Input: part model. Units: mm. Frame: model coordinates. Face numbers are marked on the shaded views. A direction names the side the tool comes from. Coordinates: 2 decimals unless noted, no trailing zeros. Order: outer loops, then holes, each group sorted by start corner. A loop starts at its lowest first (then second) coordinate and runs counter-clockwise, first axis right, second up. Notation, with made-up numbers: (-3.75, 24) -> (22.25, 24) arc R21 cw to (22.25, 36) -> close; hole circle Ø6 at (22, 6.25). An arc over 180 degrees is marked (long way). One line per item, written item: value. Start each with the question number.
from build123d import *

# Parameters (mm, degrees)
SKETCH_1_W               = 90
SKETCH_1_H               = 90
EXTRUDE_2_DEPTH          = 45
SKETCH_2_W               = 80
SKETCH_2_H               = 80
CUT_EXTRUDE_1_DEPTH      = 40
EXTRUDE_3_DEPTH          = 10
SKETCH_4_R               = 1
EXTRUDE_4_DEPTH          = 2
SKETCH_5_R               = 6
CUT_EXTRUDE_2_DEPTH      = 30
EXTRUDE_5_DEPTH          = 6
CUT_EXTRUDE_START        = -2
CUT_EXTRUDE_3_DEPTH      = 6
SKETCH_8_R               = 12.5
CUT_EXTRUDE_4_DEPTH      = 6
SKETCH_9_R               = 6
CUT_EXTRUDE_5_DEPTH      = 6
SKETCH_10_R              = 2
EXTRUDE_6_DEPTH          = 5
CUT_EXTRUDE_6_DEPTH      = 86.341501801
CUT_EXTRUDE_6_DEPTH_BACK = 86.341501801
EXTRUDE_8_DEPTH          = 5
EXTRUDE_9_REACH          = 89.762
SKETCH_13_W              = 70
SKETCH_13_H              = 5
SKETCH_14_R              = 2
SKETCH_14_W              = 3.535716984
SKETCH_14_H              = 8
EXTRUDE_10_DEPTH         = 5


with BuildPart() as part:
    # 草图1 → 凸台-拉伸2 (new body)
    with BuildSketch(Plane.XY):
        Rectangle(SKETCH_1_W, SKETCH_1_H)
    extrude(amount=EXTRUDE_2_DEPTH)

    # 草图2 → 切除-拉伸1 (cut)
    with BuildSketch(Plane.XY.offset(45)):
        Rectangle(SKETCH_2_W, SKETCH_2_H)
    extrude(amount=-CUT_EXTRUDE_1_DEPTH, mode=Mode.SUBTRACT)

    # 草图3 → 凸台-拉伸3 (add)
    with BuildSketch(Plane(origin=(0, 45, 0), x_dir=(1, 0, 0), z_dir=(0, 1, 0))):
        with BuildLine():
            Line((-15.725, -45), (15.725, -45))
            ThreePointArc((15.725, -45), (0, -29.275), (-15.725, -45))
        make_face()
    extrude(amount=EXTRUDE_3_DEPTH)

    # 草图4 → 凸台-拉伸4 (add)
    with BuildSketch(Plane(origin=(0, 55, 0), x_dir=(1, 0, 0), z_dir=(0, 1, 0))):
        with BuildLine():
            Line((-13.344644505, -28.920245738), (13.344644505, -28.920245738))
            ThreePointArc((13.344644505, -28.920245738), (16.17307163, -30.091818614), (17.344644505, -32.920245738))
            Line((17.344644505, -32.920245738), (17.344644505, -45))
            Line((17.344644505, -45), (-17.344644505, -45))
            Line((-17.344644505, -45), (-17.344644505, -32.920245738))
            ThreePointArc((-17.344644505, -32.920245738), (-16.17307163, -30.091818614), (-13.344644505, -28.920245738))
        make_face()
        with Locations(Location((13.344644505, -32.920245738, 0), (0, 0, 270))):
            Circle(SKETCH_4_R, mode=Mode.SUBTRACT)
        with Locations(Location((-13.344644505, -32.920245738, 0), (0, 0, 270))):
            Circle(SKETCH_4_R, mode=Mode.SUBTRACT)
    extrude(amount=-EXTRUDE_4_DEPTH)

    # 草图5 → 切除-拉伸2 (cut)
    with BuildSketch(Plane(origin=(0, 55, 0), x_dir=(1, 0, 0), z_dir=(0, 1, 0))):
        with Locations((0, -45)):
            Circle(SKETCH_5_R)
    extrude(amount=-CUT_EXTRUDE_2_DEPTH, mode=Mode.SUBTRACT)

    # 草图6 → 凸台-拉伸5 (add)
    with BuildSketch(Plane.ZY.offset(45)):
        with BuildLine():
            Line((45.073955752, 16.4), (45.073955752, -13.6))
            ThreePointArc((45.073955752, -13.6), (30.073955752, 1.4), (45.073955752, 16.4))
        make_face()
    extrude(amount=EXTRUDE_5_DEPTH)

    # 草图7 → 切除-拉伸3 (cut)
    with BuildSketch(Plane(origin=(0, 55, 0), x_dir=(1, 0, 0), z_dir=(0, 1, 0)).offset(CUT_EXTRUDE_START)):
        with BuildLine():
            Line((-12.5, -45), (12.5, -45))
            ThreePointArc((12.5, -45), (0, -32.5), (-12.5, -45))
        make_face()
    extrude(amount=-CUT_EXTRUDE_3_DEPTH, mode=Mode.SUBTRACT)

    # 草图8 → 切除-拉伸4 (cut)
    with BuildSketch(Plane.ZY.offset(51)):
        with Locations((45.073955752, 1.4)):
            Circle(SKETCH_8_R)
    extrude(amount=-CUT_EXTRUDE_4_DEPTH, mode=Mode.SUBTRACT)

    # 草图9 → 切除-拉伸5 (cut)
    with BuildSketch(Plane.ZY.offset(45)):
        with Locations((45, 1.4)):
            Circle(SKETCH_9_R)
    extrude(amount=-CUT_EXTRUDE_5_DEPTH, mode=Mode.SUBTRACT)

    # 草图10 → 凸台-拉伸6 (add)
    # profile 1 of 4: a face of its own
    with BuildSketch(Plane.XY.offset(45)):
        with BuildLine():
            Line((-47.5, 45), (-42.902808048, 45))
            Line((-42.902808048, 45), (-42.902808048, 37))
            Line((-42.902808048, 37), (-47.5, 37))
            ThreePointArc((-47.5, 37), (-51.5, 41), (-47.5, 45))
        make_face()
        with Locations((-47.5, 41)):
            Circle(SKETCH_10_R, mode=Mode.SUBTRACT)
    # profile 2 of 4: a face of its own
    with BuildSketch(Plane.XY.offset(45)):
        with BuildLine():
            Line((-47.5, -45), (-42.902808048, -45))
            Line((-42.902808048, -45), (-42.902808048, -37))
            Line((-42.902808048, -37), (-47.5, -37))
            ThreePointArc((-47.5, -37), (-51.5, -41), (-47.5, -45))
        make_face()
        with Locations((-47.5, -41)):
            Circle(SKETCH_10_R, mode=Mode.SUBTRACT)
    # profile 3 of 4: a face of its own
    with BuildSketch(Plane.XY.offset(45)):
        with BuildLine():
            Line((42.460881889, 45), (42.460881889, 37))
            Line((42.460881889, 37), (47.5, 37))
            ThreePointArc((47.5, 37), (51.5, 41), (47.5, 45))
            Line((47.5, 45), (42.460881889, 45))
        make_face()
        with Locations((47.5, 41)):
            Circle(SKETCH_10_R, mode=Mode.SUBTRACT)
    # profile 4 of 4: a face of its own
    with BuildSketch(Plane.XY.offset(45)):
        with BuildLine():
            Line((41.065096799, -37), (41.065096799, -45))
            Line((41.065096799, -45), (47.5, -45))
            ThreePointArc((47.5, -45), (51.5, -41), (47.5, -37))
            Line((47.5, -37), (41.065096799, -37))
        make_face()
        with Locations((47.5, -41)):
            Circle(SKETCH_10_R, mode=Mode.SUBTRACT)
    extrude(amount=-EXTRUDE_6_DEPTH)

    # 草图11 → 切除-拉伸6 (cut, two sides: drawn at the far end of the back side and taken through both)
    with BuildSketch(Plane.XY.offset(5).offset(-CUT_EXTRUDE_6_DEPTH_BACK)):
        Polygon((25, 25), (25, 60.762211799), (85.89289348, 60.762211799), (85.89289348, -73.939659246), (-86.710921037, -73.939659246), (-86.710921037, -25), (-25, -25), (25, -25), align=None)
    extrude(amount=CUT_EXTRUDE_6_DEPTH + CUT_EXTRUDE_6_DEPTH_BACK, mode=Mode.SUBTRACT)

    # 草图12 → 凸台-拉伸8 (add)
    with BuildSketch(Plane(origin=(25, 0, 0), x_dir=(0, 0, -1), z_dir=(1, 0, 0))):
        Polygon((-45, 40), (-45, -25), (-5, -25), (0, -25), (0, 45), (-45, 45), align=None)
    extrude(amount=-EXTRUDE_8_DEPTH)

    # 草图13 → 凸台-拉伸9 (add, up to next)
    with BuildSketch(Plane.XY.offset(45), mode=Mode.PRIVATE) as extrude_9_sk1:
        with Locations((-10, -22.5)):
            Rectangle(SKETCH_13_W, SKETCH_13_H)
    extrude_9_tool1 = extrude(extrude_9_sk1.sketch, amount=-EXTRUDE_9_REACH, mode=Mode.PRIVATE) - part.part
    add(extrude_9_tool1.solids().sort_by_distance((-10, -22.5, 45))[0])

    # 草图14 → 凸台-拉伸10 (add)
    # profile 1 of 5: a face of its own
    with BuildSketch(Plane.XY.offset(45)):
        with BuildLine():
            Line((27.5, 45), (25, 45))
            Line((25, 45), (25, 37))
            Line((25, 37), (27.5, 37))
            ThreePointArc((27.5, 37), (31.5, 41), (27.5, 45))
        make_face()
        with Locations((27.5, 41)):
            Circle(SKETCH_14_R, mode=Mode.SUBTRACT)
    # profile 2 of 5: a face of its own
    with BuildSketch(Plane.XY.offset(45)):
        with Locations((-43.232141508, -21)):
            Rectangle(SKETCH_14_W, SKETCH_14_H)
    # profile 3 of 5: a face of its own
    with BuildSketch(Plane.XY.offset(45)):
        with Locations((23.232141508, -21)):
            Rectangle(SKETCH_14_W, SKETCH_14_H)
    # profile 4 of 5: a face of its own
    with BuildSketch(Plane.XY.offset(45)):
        with BuildLine():
            Line((27.5, -17), (25, -17))
            Line((25, -17), (25, -25))
            Line((25, -25), (27.5, -25))
            ThreePointArc((27.5, -25), (31.5, -21), (27.5, -17))
        make_face()
        with Locations((27.5, -21)):
            Circle(SKETCH_14_R, mode=Mode.SUBTRACT)
    # profile 5 of 5: a face of its own
    with BuildSketch(Plane.XY.offset(45)):
        with BuildLine():
            Line((-47.5, -25), (-45, -25))
            Line((-45, -25), (-45, -17))
            Line((-45, -17), (-47.5, -17))
            ThreePointArc((-47.5, -17), (-51.5, -21), (-47.5, -25))
        make_face()
        with Locations((-47.5, -21)):
            Circle(SKETCH_14_R, mode=Mode.SUBTRACT)
    extrude(amount=-EXTRUDE_10_DEPTH)


solid = part.part
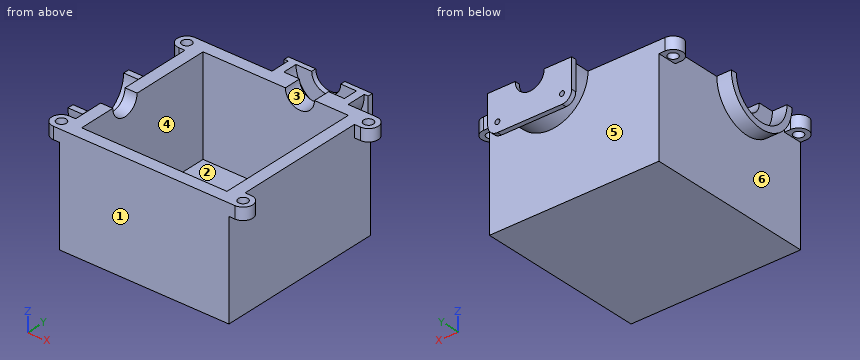
1) Ray query, line 1 along Y through (x, z) = (12, 42.5); line 2 along Y through (x, z) = (-47, 42); line 3 along X through (y, z) = (25, 12). Return the intervals inside material, ascending. Write a range as from..to.
2) Section query D-D, the plane y = 24. Return the cut outline in (x, z).
3) Pin query (flat end, axial travel): pin 1 Ø2.5 at (x, y) = (27.5, -21) entering from +Z; pin 2 Ø12 at (y, z) = (-6, 11) entering from +X; pin 3 Ø5 at (x, y) = (-12, 31) entering from +Z; pin 4 Ø5 at (x, y) = (29, -20.5) entering from -Z. Return the tip coordinate at first contact, or that it passes through.
4) Section query C-C, the plane z = 27.5. Return the cut outline in (x, y), plus the area to 3 significant figures.
5) Section query B-B, the plane x = -27. Return the cut outline in (y, z).
6) Mould query, pull axis X, two halves, no side actions, for the marked faces 4, 5 and 6. Classes: +X half, -X half, draft (parallel to the pull), parting line (faces both ways), or undercut.
7) Section query A-A, the plane y = 41. Return the cut outline in (x, z).
8) Access query for the marked faces 1, 2 and 3. Directions: +Z, -Z, +X, -X, +Y, -Y. A direction counts if a zero-diameter tool reaches every point of the face in a straight line with its end or side. Return the directions, or none.
Entries:
1. line 1: y = -25..-20, 40..47, 53..55
1. line 2: y = -25..-22.94, -19.06..-17, -13.28..-10.72, 13.52..16.08, 37..39.06, 42.94..45
1. line 3: x = -45..-40, 20..25
2. outline: (-45, 0) -> (25, 0) -> (25, 45) -> (20, 45) -> (20, 5) -> (-40, 5) -> (-40, 45) -> (-45, 45) -> close
3. pin 1: passes through
3. pin 2: stops at x = 25
3. pin 3: stops at z = 5
3. pin 4: stops at z = 40
4. outline: (-45, -25) -> (25, -25) -> (25, 45) -> (-45, 45) -> close; hole (-40, -20) -> (20, -20) -> (20, 40) -> (-40, 40) -> close
4. area: 1,300 mm2
5. outline: (-25, 0) -> (45, 0) -> (45, 45) -> (40, 45) -> (40, 5) -> (-20, 5) -> (-20, 45) -> (-25, 45) -> close
6. face 4: undercut
6. face 5: draft
6. face 6: -X half
7. outline: (-51.5, 40) -> (-49.5, 40) -> (-49.5, 45) -> (-51.5, 45) -> close; (-45.5, 40) -> (-45, 40) -> (-45, 0) -> (25, 0) -> (25, 40) -> (25.5, 40) -> (25.5, 45) -> (6, 45) arc R6 cw to (-6, 45) -> (-45.5, 45) -> close; (29.5, 40) -> (31.5, 40) -> (31.5, 45) -> (29.5, 45) -> close
8. face 1: +Z, -Z, +X, -X, -Y
8. face 2: +Z
8. face 3: +Z, +Y
